Can you work these out from the model? Positions are in its coordinate system, mm. A direction names the side the tool comes from. Round coordinates to 2 decimals unless told otherwise and drop trailing zeros. Write each loop counter-clockwise with the first axis right and the second up, starting at its lowest first coordinate (ties: lowest second). Pieces come first, ordered by that corner, then holes.
Q1. Please list where these lines run through material, in increasing order: line 1 along Z through (x, y) = (1.5, -7.5); line 2 along Y through (x, z) = (4.25, 11.25); line 3 along Z through (x, y) = (11, -0.5).
Q2. I'm going to push flat-ended pins straight in: pin 1 Ø1 at (x, y) = (8, -2.5) entering from +Z; pin 2 Ø1.6 at (x, z) = (11, 8) entering from -Y; pin 3 Ø1.2 at (x, y) = (5, -0.5) entering from +Z. Where does each tip first touch, or does it pass through?
Q3. If we section it at D-D (z = 12.5): Please give me the cut outline in (x, y), plus the area to 3 significant figures.
Q4. If we section it at A-A (y = -0.25): Please give me the cut outline in (x, z), plus the area to 3 significant figures.
Q5. If we section it at C-C (x = 7.5): Please give me the cut outline in (y, z), plus the area to 3 significant figures.
Q6. We'd pull the mould along Z, two halves only. Please class faces 4 (the flat face through (8, -4, 0)), 5 (the flat face through (0, -4, 2)), 6 (the cylindrical face through (8.42, -2.73, 12.4)): +Z half, -Z half, draft (parallel to the pull), parting line (faces both ways), or undercut.
Q7. For faces 1 (the flat face through (6.037, -1, 13)), 2 (the flat face through (11, -1, 12.246)), 3 (the flat face through (11, -1.502, 8)), which set-ups out of +Z, -Z, +X, -X, +Y, -Y let a thin tool reach every point of the face, with its end or its side?
Q8. If we section it at B-B (y = -3): Please give me the cut outline in (x, z), plus the area to 3 significant figures.
from build123d import *

# Parameters (mm, degrees)
F0_W     = 15.8174857497
F0_H     = 3.4455414861
F1_DEPTH = 7.8
F3_DEPTH = 8.8
F4_W     = 3.7536188029
F4_H     = 1.5020088758
F5_DEPTH = 2.37
F6_R     = 1.163766632
F7_DEPTH = 2.5


with BuildPart() as f1:
    # F0 (on Front) → F1 (new body)
    with BuildSketch(Plane.XZ):
        with Locations((7.9087428749, 1.7227707431)):
            Rectangle(F0_W, F0_H)
    extrude(amount=F1_DEPTH)

    # F2 (on face) → F3 (join)
    with BuildSketch(Plane.XY.offset(3.4455414861)):
        Polygon((11.810105294, -1.5020088758), (11.810105294, 0), (4.0005231276, 0), (4.0005231276, -1.5020088758), (6.037354935, -1.5020088758), (9.7909737378, -1.5020088758), align=None)
        with BuildLine():
            ThreePointArc((6.037354935, -1.5020088758), (7.9141643364, -2.7745180875), (9.7909737378, -1.5020088758))
            Line((9.7909737378, -1.5020088758), (6.037354935, -1.5020088758))
        make_face()
    extrude(amount=F3_DEPTH)

    # F4 (on face) → F5 (join)
    with BuildSketch(Plane.XY.offset(12.2455414861)):
        with Locations((7.9141643364, -0.7510044379)):
            Rectangle(F4_W, F4_H)
    extrude(amount=F5_DEPTH)

    # F6 (on face) → F7 (join)
    with BuildSketch(Plane.XZ.offset(1.5020088758)):
        with Locations((7.8803384677, 13.4305414861)):
            Circle(F6_R)
    extrude(amount=F7_DEPTH)


solid = f1.part
A:
1. line 1: z = 0 to 3.45
1. line 2: y = -1.5 to 0
1. line 3: z = 0 to 12.25
2. pin 1: stops at z = 14.59
2. pin 2: stops at y = -1.5
2. pin 3: stops at z = 12.25
3. outline: (6.04, -1.5) - (7.18, -1.5) - (7.18, -4) - (8.58, -4) - (8.58, -1.5) - (9.79, -1.5) - (9.79, 0) - (6.04, 0) - close
3. area: 9.13 mm2
4. outline: (0, 0) - (15.82, 0) - (15.82, 3.45) - (11.81, 3.45) - (11.81, 12.25) - (9.79, 12.25) - (9.79, 14.62) - (6.04, 14.62) - (6.04, 12.25) - (4, 12.25) - (4, 3.45) - (0, 3.45) - close
4. area: 132 mm2
5. outline: (-7.8, 0) - (0, 0) - (0, 14.62) - (-1.5, 14.62) - (-1.5, 14.53) - (-4, 14.53) - (-4, 12.33) - (-1.5, 12.33) - (-1.5, 12.25) - (-2.73, 12.25) - (-2.73, 3.45) - (-7.8, 3.45) - close
5. area: 60.0 mm2
6. face 4: -Z half
6. face 5: draft
6. face 6: undercut
7. face 1: +Z, -X, +Y, -Y
7. face 2: +Z, +X, +Y, -Y
7. face 3: +Z, +X, -Y
8. outline: (0, 0) - (15.82, 0) - (15.82, 3.45) - (0, 3.45) - close; circle Ø2.33 at (7.88, 13.43)
8. area: 58.8 mm2
